The listing builds one solid part. Answer for the finished solid, in the listing's coordinates (mm). Face numbers are marked on the shaded views. A direction names the side the tool comes from. Coordinates: 2 decimals unless noted, no trailing zeros. Write each loop counter-clockwise with the first axis right and the second up, starting at its lowest first coordinate (ties: lowest second). Pieces come first, ordered by that corner, then holes.
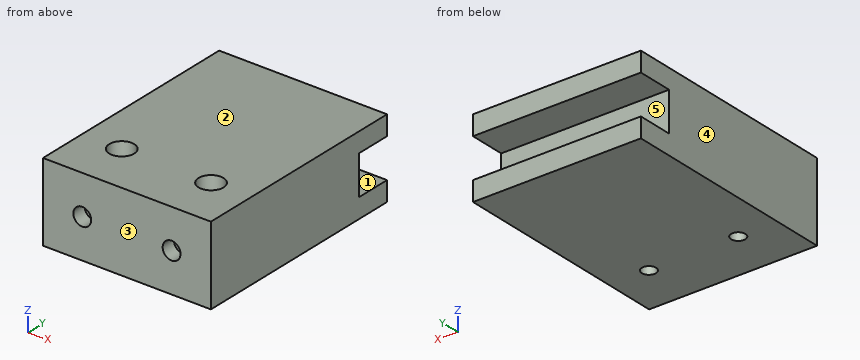
from build123d import *

# Parameters (mm, degrees)
SKETCH1_W               = 47
SKETCH1_H               = 62.5
BOSS_EXTRUDE1_DEPTH     = 22
SKETCH2_W               = 60
SKETCH2_H               = 11
CUT_EXTRUDE1_DEPTH      = 10
CUT_EXTRUDE2_DEPTH      = 82.235767984
CUT_EXTRUDE2_DEPTH_BACK = 82.235767984
SKETCH3_R               = 2
CUT_EXTRUDE3_DEPTH      = 82.235767984
CUT_EXTRUDE3_DEPTH_BACK = 4
SKETCH3_3_R             = 3.5
SKETCH3_3_R_2           = 2
SKETCH4_R               = 1.5
CUT_EXTRUDE6_DEPTH      = 13
SKETCH4_3_R             = 2.5
SKETCH4_3_R_2           = 1.5
CUT_EXTRUDE7_DEPTH      = 4


with BuildPart() as part:
    # Sketch1 → Boss-Extrude1 (new body)
    with BuildSketch(Plane.XY):
        with Locations((-23.5, 31.25)):
            Rectangle(SKETCH1_W, SKETCH1_H)
    extrude(amount=BOSS_EXTRUDE1_DEPTH)

    # Sketch2 → Cut-Extrude1 (cut)
    with BuildSketch(Plane(origin=(0, 62.5, 0), x_dir=(1, 0, 0), z_dir=(0, 1, 0))):
        with Locations((-23.5, -11)):
            Rectangle(SKETCH2_W, SKETCH2_H)
    extrude(amount=-CUT_EXTRUDE1_DEPTH, mode=Mode.SUBTRACT)

    # Sketch3 → Cut-Extrude2 (cut, two sides: drawn at the far end of the back side and taken through both)
    with BuildSketch(Plane.XY.offset(22).offset(-CUT_EXTRUDE2_DEPTH_BACK)):
        with Locations((-36, 14)):
            Circle(SKETCH3_R)
        with Locations((-11, 14)):
            Circle(SKETCH3_R)
    extrude(amount=CUT_EXTRUDE2_DEPTH + CUT_EXTRUDE2_DEPTH_BACK, mode=Mode.SUBTRACT)

    # Sketch3_3 → Cut-Extrude3 (cut, two sides: drawn at the far end of the back side and taken through both)
    # profile 1 of 2: a face of its own
    with BuildSketch(Plane.XY.offset(22).offset(-CUT_EXTRUDE3_DEPTH_BACK)):
        with Locations(Location((-36, 14, 0), (0, 0, 180))):
            Circle(SKETCH3_3_R)
        with Locations((-36, 14)):
            Circle(SKETCH3_3_R_2, mode=Mode.SUBTRACT)
    # profile 2 of 2: a face of its own
    with BuildSketch(Plane.XY.offset(22).offset(-CUT_EXTRUDE3_DEPTH_BACK)):
        with Locations(Location((-11, 14, 0), (0, 0, 180))):
            Circle(SKETCH3_3_R)
        with Locations((-11, 14)):
            Circle(SKETCH3_3_R_2, mode=Mode.SUBTRACT)
    extrude(amount=CUT_EXTRUDE3_DEPTH + CUT_EXTRUDE3_DEPTH_BACK, mode=Mode.SUBTRACT)

    # Sketch4 → Cut-Extrude6 (cut)
    with BuildSketch(Plane.XZ):
        with Locations(Location((-11, 11, 0), (0, 0, 270))):
            Circle(SKETCH4_R)
        with Locations(Location((-36, 11, 0), (0, 0, 270))):
            Circle(SKETCH4_R)
    extrude(amount=-CUT_EXTRUDE6_DEPTH, mode=Mode.SUBTRACT)

    # Sketch4_3 → Cut-Extrude7 (cut)
    # profile 1 of 2: a face of its own
    with BuildSketch(Plane.XZ):
        with Locations((-36, 11)):
            Circle(SKETCH4_3_R)
        with Locations(Location((-36, 11, 0), (0, 0, 270))):
            Circle(SKETCH4_3_R_2, mode=Mode.SUBTRACT)
    # profile 2 of 2: a face of its own
    with BuildSketch(Plane.XZ):
        with Locations((-11, 11)):
            Circle(SKETCH4_3_R)
        with Locations(Location((-11, 11, 0), (0, 0, 270))):
            Circle(SKETCH4_3_R_2, mode=Mode.SUBTRACT)
    extrude(amount=-CUT_EXTRUDE7_DEPTH, mode=Mode.SUBTRACT)


solid = part.part
1. Find the intervals of material crossed by L1, parallel to X at y = 14, z = 9.25; L2, parallel to X at y = 14, z = 19.9; L3, parallel to Z at x = -36, y = 1.8, in increasing order.
Results found:
L1: x = -47 to -38, -34 to -13, -9 to 0
L2: x = -47 to -39.5, -32.5 to -14.5, -7.5 to 0
L3: z = 0 to 8.5, 13.5 to 22
2. Section C-C on y = 57 is taken. Give the vertices of the cut face in (x, z), then the cut area to 3 significant figures.
Results found:
outline: (-47, 0) - (0, 0) - (0, 5.5) - (-47, 5.5) - close; (-47, 16.5) - (0, 16.5) - (0, 22) - (-47, 22) - close
area: 517 mm2
3. Section D-D on z = 19.5 is taken. Give the vertices of the cut face in (x, y).
Results found:
outline: (-47, 0) - (0, 0) - (0, 62.5) - (-47, 62.5) - close; hole circle Ø7 at (-36, 14); hole circle Ø7 at (-11, 14)
4. Section A-A on x = -36 is taken. Give the vertices of the cut face in (y, z).
Results found:
outline: (0, 0) - (12, 0) - (12, 9.5) - (4, 9.5) - (4, 8.5) - (0, 8.5) - close; (0, 13.5) - (4, 13.5) - (4, 12.5) - (12, 12.5) - (12, 18) - (10.5, 18) - (10.5, 22) - (0, 22) - close; (16, 0) - (62.5, 0) - (62.5, 5.5) - (52.5, 5.5) - (52.5, 16.5) - (62.5, 16.5) - (62.5, 22) - (17.5, 22) - (17.5, 18) - (16, 18) - close
5. Flat-ended cylindrical pins translate along their axes: P1, Ø1.5, axis at x = -35, z = 12, coming from the -Y side; P2, Ø2, axis at x = -24.5, z = 9, coming from the +Y side; P3, Ø6.5, axis at x = -11, y = 14, coming from the +Z side. Find the tip coordinate at first contact, or state that the pin passes through.
Results found:
P1: stops at y = 4
P2: stops at y = 52.5
P3: stops at z = 18
6. A tool of negligible diameter and unlimited length cuts with its end or side. For the marked faces 4 and 5, from which of +Z, -Z, +X, -X, +Y, -Y can it reach the whole face along a straight path? Write none if from no direction.
Results found:
face 4: +Z, -Z, -X, +Y, -Y
face 5: +X, -X, +Y
7. For a pull along Z with two mould halves and no side action, classify the marked faces 1, 2 and 3 as pulls with the +Z half, pulls with the -Z half, needs draft (parallel to the pull), parting line crosses it, or undercut.
Results found:
face 1: undercut
face 2: pulls with the +Z half
face 3: needs draft
8. Section B-B on y = 14 is taken. Give the vertices of the cut face in (x, z).
Results found:
outline: (-47, 0) - (-38, 0) - (-38, 18) - (-39.5, 18) - (-39.5, 22) - (-47, 22) - close; (-34, 0) - (-13, 0) - (-13, 18) - (-14.5, 18) - (-14.5, 22) - (-32.5, 22) - (-32.5, 18) - (-34, 18) - close; (-9, 0) - (0, 0) - (0, 22) - (-7.5, 22) - (-7.5, 18) - (-9, 18) - close
